The drawing under review shows one solid part. Ordinate dimensions are in mm from its lowest x, y, z. A direction names the side the tool comes from. Round coordinates to 2 decimals unless told otherwise and drop trailing zeros. Write each loop counter-clockwise with the first axis right and the second up, starting at its lowest first coordinate (ties: lowest second). Pieces come first, ordered by that corner, then holes. Notation, with made-up numbers: M 21,-13.5 L 72,-13.5 A28 cw 72,16.5 Z; hole C 65,-6 d3. An arc over 180 degrees is marked long. Write item = value, one per line. Start each with the question number.
Item 1: Take a section at C-C, the plane z = 25.5. Give the boundary of the cut face in (x, y).
Item 2: For pin 1 Ø4 at (y, z) = (6.5, 27.5) entering from -X; pin 2 Ø4 at (x, y) = (162.5, 5) entering from -Z, all flat-tipped, find the tip position at first contact; note any pin that passes through.
Item 3: Take a section at A-A, the plane y = 9. Give the boundary of the cut face in (x, z), plus the area to 3 significant figures.
Item 4: The part is to be moulded in two halves that separate along Z. For the marked faces 1, 2, 3 and 4, say which applies: +Z half, -Z half, draft (parallel to the pull), parting line (faces both ways), or undercut.
Item 5: Take a section at B-B, the plane x = 179. Give the boundary of the cut face in (y, z), plus the area to 3 significant figures.
Item 6: To check wall thickness, follow line 1 along Z through (x, y) = (179, 10); line 2 along Z through (x, y) = (217, 5); line 3 along Y through (x, z) = (65.5, 21). State the ranges of each line that lie inside material, in increasing order.
Item 7: Tool access review of the marked faces 5 and 6: name each direction out of +Z, -Z, +X, -X, +Y, -Y from which nothing blocks a thin tool from reaching the whole face with its end or side.
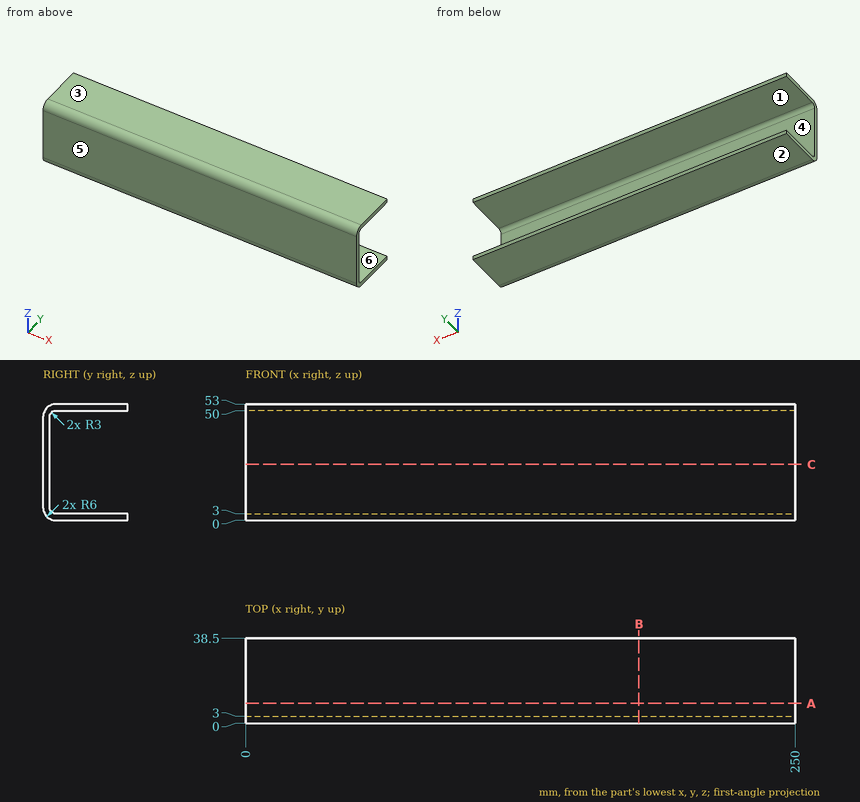
Response values:
q1.outline = M 0,0 L 250,0 L 250,3 L 0,3 Z
q2.pin_1 = through
q2.pin_2 = 0
q3.outline = M 0,0 L 250,0 L 250,3 L 0,3 Z; M 0,50 L 250,50 L 250,53 L 0,53 Z
q3.area = 1,500 mm2
q4.face_1 = undercut
q4.face_2 = -Z half
q4.face_3 = +Z half
q4.face_4 = undercut
q5.outline = M 0,6 A6 ccw 6,0 L 38.5,0 L 38.5,3 L 6,3 A3 cw 3,6 L 3,47 A3 cw 6,50 L 38.5,50 L 38.5,53 L 6,53 A6 ccw 0,47 Z
q5.area = 360 mm2
q6.line_1 = 0 to 3, 50 to 53
q6.line_2 = 0.08 to 3.17, 49.83 to 52.92
q6.line_3 = 0 to 3
q7.face_5 = +Z, -Z, +X, -X, -Y
q7.face_6 = +X, -X, +Y
